The model under review builds one solid part; all positions refer to its coordinate system, in mm. Face numbers are marked on the shaded views. A direction names the side the tool comes from. Round coordinates to 2 decimals unless told otherwise and drop trailing zeros. Write each loop counter-clockwise with the first axis right and the second up, starting at its lowest first coordinate (ties: lowest second). Pieces come first, ordered by that corner, then holes.
Item 1: Machinability: for the marked faces 4, 5, 6, 7 and 8, which of the approach directions +Z, -Z, +X, -X, +Y, -Y give a long, thin tool a straight path to every point of the face, cutting with its end or side? Answer none if there is none.
Item 2: To check wall thickness, follow L1, parallel to X at y = -4.5, z = 30.6; L2, parallel to Z at x = 5.75, y = 3.5 (3 decimals); L3, parallel to Y at x = 13.75, z = 22.5 (3 decimals). State the ranges of each line that lie inside material, in increasing order.
Item 3: Draft analysis for pull direction Z (two halves, no side actions). For the marked faces 1, 2 and 3, state which applies: +Z half, -Z half, draft (parallel to the pull), parting line (faces both ways), or undercut.
Item 4: Add section B-B (y = 5). Give the boundary of the cut face in (x, z) (3 decimals), plus the area to 3 significant figures.
Item 5: Add section C-C (y = -8). Give the boundary of the cut face in (x, z).
Item 6: Clearance check with flat-ended pins moving along their axes: pin 1 Ø10 at (x, z) = (10, -30.5) entering from -Y; pin 2 Ø4 at (x, z) = (4.5, 10) entering from -Y; pin 3 Ø3 at (x, z) = (7.5, -5) entering from +Y. State where each tip first meets the part, or that it passes through.
Item 7: Add section D-D (x = 17). Give the boundary of the cut face in (y, z) (3 decimals).
Item 8: Add section A-A (z = -30.6). Give the boundary of the cut face in (x, y) (3 decimals).
```python
from build123d import *

# Parameters (mm, degrees)
BOSS_EXTRUDE1_DEPTH = 20
CUT_EXTRUDE1_REACH  = 57.463
SKETCH3_R           = 4


with BuildPart() as part:
    # Sketch2 → Boss-Extrude1 (new body)
    with BuildSketch(Plane(origin=(0, 0, 0), x_dir=(0, 0, -1), z_dir=(1, 0, 0))):
        with BuildLine():
            Line((-18.601140422, -10.16), (-38.601140422, -10.16))
            Line((-38.601140422, -10.16), (-38.601140422, 0))
            Line((-38.601140422, 0), (-38.601140422, 13.245))
            Line((-38.601140422, 13.245), (-11.035, 13.245))
            Line((-11.035, 13.245), (-11.035, 0))
            ThreePointArc((-11.035, 0), (0, -11.035), (11.035, 0))
            Line((11.035, 0), (11.035, 13.245))
            Line((11.035, 13.245), (38.601140422, 13.245))
            Line((38.601140422, 13.245), (38.601140422, -10.16))
            Line((38.601140422, -10.16), (18.601140422, -10.16))
            ThreePointArc((18.601140422, -10.16), (0, -21.195), (-18.601140422, -10.16))
        make_face()
    extrude(amount=BOSS_EXTRUDE1_DEPTH)

    # Sketch3 → Cut-Extrude1 (cut, up to next)
    with BuildSketch(Plane(origin=(0, 13.245, 0), x_dir=(1, 0, 0), z_dir=(0, 1, 0)), mode=Mode.PRIVATE) as cut_extrude1_sk1:
        with Locations(Location((10, -30.6, 0), (0, 0, 270))):
            Circle(SKETCH3_R)
    cut_extrude1_tool1 = extrude(cut_extrude1_sk1.sketch, amount=-CUT_EXTRUDE1_REACH, mode=Mode.PRIVATE) & part.part
    # Sketch3 → Cut-Extrude1 (cut, up to next)
    with BuildSketch(Plane(origin=(0, 13.245, 0), x_dir=(1, 0, 0), z_dir=(0, 1, 0)), mode=Mode.PRIVATE) as cut_extrude1_sk2:
        with Locations(Location((10, 30.6, 0), (0, 0, 270))):
            Circle(SKETCH3_R)
    cut_extrude1_tool2 = extrude(cut_extrude1_sk2.sketch, amount=-CUT_EXTRUDE1_REACH, mode=Mode.PRIVATE) & part.part
    add(cut_extrude1_tool1.solids().sort_by_distance((10, 13.245, 30.6))[0], mode=Mode.SUBTRACT)
    add(cut_extrude1_tool2.solids().sort_by_distance((10, 13.245, -30.6))[0], mode=Mode.SUBTRACT)


solid = part.part
```
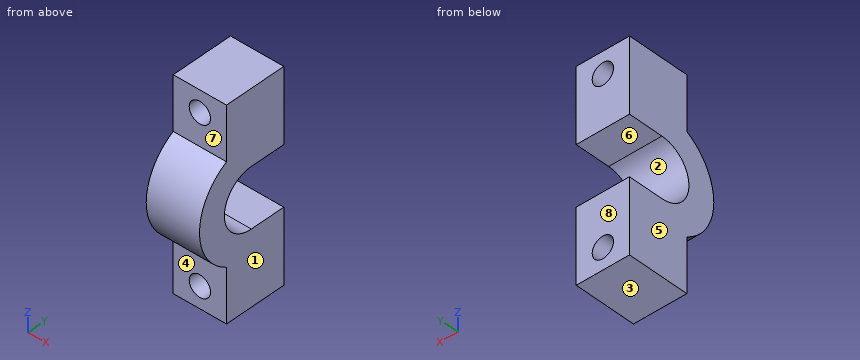
Numbers:
1. face 4: -Z, +X, -X, -Y
1. face 5: +Z, -Z, -X, +Y, -Y
1. face 6: +X, -X, +Y
1. face 7: +Z, +X, -X, -Y
1. face 8: +Z, -Z, +X, -X, +Y
2. L1: x = 0 to 6, 14 to 20
2. L2: z = -38.601 to -11.035, 11.035 to 38.601
2. L3: y = -10.16 to 13.245
3. face 1: draft
3. face 2: undercut
3. face 3: -Z half
4. outline: (0, -38.601) - (20, -38.601) - (20, -11.035) - (0, -11.035) - close; (0, 11.035) - (20, 11.035) - (20, 38.601) - (0, 38.601) - close; hole circle Ø8 at (10, -30.6); hole circle Ø8 at (10, 30.6)
4. area: 1,000 mm2
5. outline: (0, -38.6) - (20, -38.6) - (20, -7.6) - (0, -7.6) - close; (0, 7.6) - (20, 7.6) - (20, 38.6) - (0, 38.6) - close; hole circle Ø8 at (10, -30.6); hole circle Ø8 at (10, 30.6)
6. pin 1: stops at y = -10.16
6. pin 2: stops at y = -19.63
6. pin 3: stops at y = -8.92
7. outline: (-10.16, -38.601) - (13.245, -38.601) - (13.245, -11.035) - (0, -11.035) arc R11.035 cw to (0, 11.035) - (13.245, 11.035) - (13.245, 38.601) - (-10.16, 38.601) - (-10.16, 18.601) arc R21.195 ccw to (-10.16, -18.601) - close
8. outline: (0, -10.16) - (6, -10.16) - (6, 13.245) - (0, 13.245) - close; (14, -10.16) - (20, -10.16) - (20, 13.245) - (14, 13.245) - close
